Drawing for the job (mm, zero at the part's lowest x, y, z). A direction names the side the tool comes from. Round coordinates to 2 decimals unless told otherwise and drop trailing zeros. Write each loop counter-clockwise with the first axis right and the second up, starting at its lowest first coordinate (ties: lowest second). Pieces come first, ordered by that corner, then holes.
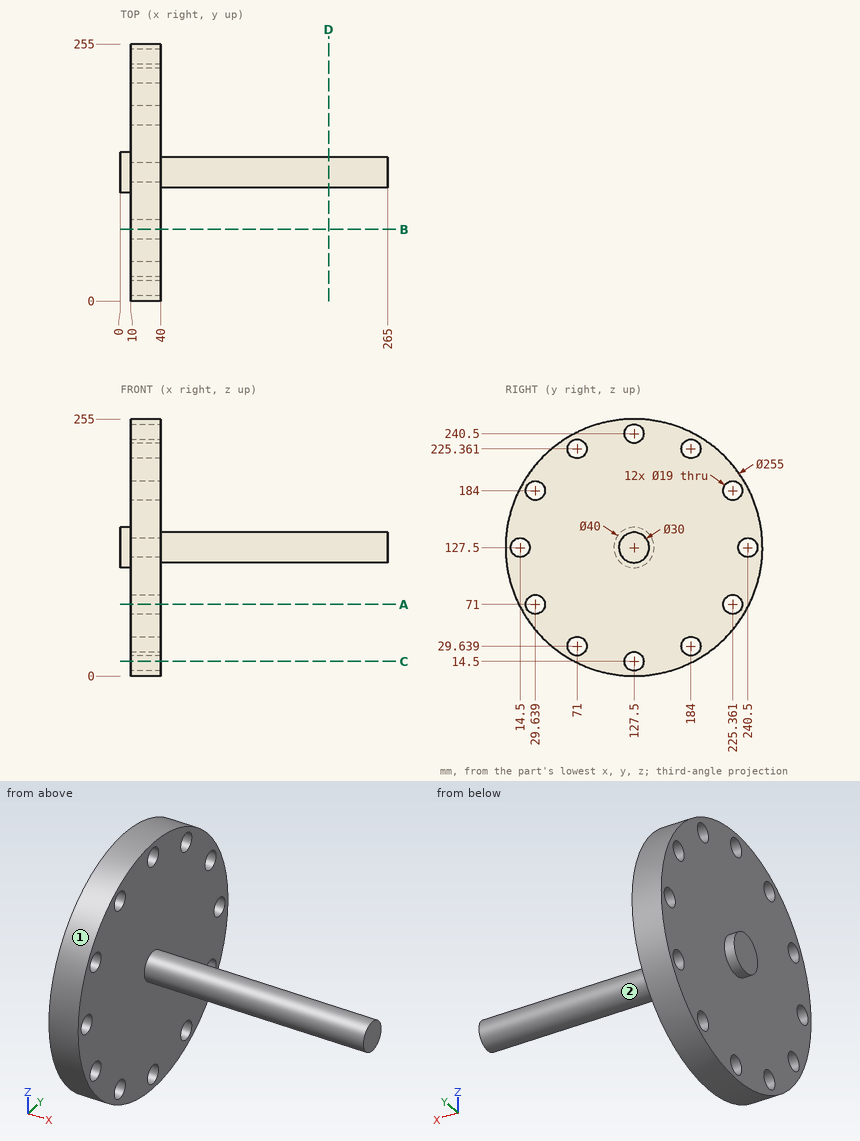
1) Flat gauge pins, fed straight in: pin 1 Ø17 at (y, z) = (184, 225.36) entering from +X (3 decimals); pin 2 Ø6 at (x, y) = (183, 126) entering from +Z; pin 3 Ø4 at (y, z) = (128, 178) entering from -X; pin 4 Ø5 at (x, y) = (30.5, 155) entering from +Z (3 decimals). Where does each tip first touch, or does it go through?
2) Cut at D-D on x = 206.5. List the corners of the cut face in (y, z), and give its area (3 significant figures).
3) Cut at C-C on z = 14.5. List the corners of the cut face in (x, y).
4) Cut at A-A on z = 71. List the corners of the cut face in (x, y).
5) Wall check: probe 1 along Y at (x, z) = (22, 127); probe 2 along Y at (x, z) = (15.5, 223) (1 decimal); probe 3 along Y at (x, z) = (192, 128.5). Give the ranges that are in metal, low to high.
6) Which spindle directions (+Z, -Z, +X, -X, +Y, -Y) get a long thin tool onto all of the face, cutting with end or side? Do the marked faces 1 and 2. Say none if no direction does.
Result sheet:
1. pin 1: passes through
1. pin 2: stops at z = 142.5
1. pin 3: stops at x = 10
1. pin 4: stops at z = 252.525
2. outline: circle Ø30 at (127.5, 127.5)
2. area: 707 mm2
3. outline: (10, 68.45) - (40, 68.45) - (40, 118) - (10, 118) - close; (10, 137) - (40, 137) - (40, 186.55) - (10, 186.55) - close
4. outline: (10, 13.2) - (40, 13.2) - (40, 20.14) - (10, 20.14) - close; (10, 39.14) - (40, 39.14) - (40, 215.86) - (10, 215.86) - close; (10, 234.86) - (40, 234.86) - (40, 241.8) - (10, 241.8) - close
5. probe 1: y = 0 to 5.01, 23.99 to 231.01, 249.99 to 255
5. probe 2: y = 43 to 61.8, 80.2 to 174.8, 193.2 to 212
5. probe 3: y = 112.53 to 142.47
6. face 1: +X, -X
6. face 2: +X
